Could you check a few things on this drawing? It's one solid part, dimensions in mm from its lowest x, y, z. A direction names the side the tool comes from. Round coordinates to 2 decimals unless told otherwise and drop trailing zeros. Write each loop counter-clockwise with the first axis right and the second up, starting at its lowest first coordinate (ties: lowest second). Pieces come first, ordered by that corner, then holes. Notation, with made-up numbers: (60, 10.5) -> (92, 10.5) arc R3 cw to (92, 14.5) -> close; hole circle Ø9 at (-19.75, -36). An arc over 180 degrees is marked (long way). Put each result on its own line as item: value. Start each with the question number.
1) Which directions (+Z, -Z, +X, -X, +Y, -Y) give clear straight access to the entire face, cutting with the end or side of a thin tool? Please do the marked faces 1 and 2.
2) I want a section at D-D, the plane y = 8.5. List the corners of the cut face in (x, z) for me (1 decimal).
3) I want a section at A-A, the plane y = 14. List the corners of the cut face in (x, z) for me (1 decimal).
4) If I drill on line 1 along Z through (x, y) = (29, 6.5); line 2 along Z through (x, y) = (22, 17.5) (1 decimal); line 3 along X through (y, z) = (15.5, 23) (1 decimal), over which ranges is the centre line in solid material (lowest first)? Write a range as [from, to].
5) Will these pins go through, and if not, where does the flat tip stop? P1, Ø10, axis at y = 4.5, z = 47.5, coming from the +X side; P2, Ø3, axis at y = 15.5, z = 24.5, coming from the +X side; P3, Ø3, axis at x = 30.5, y = 14.5, coming from the -Z side.
6) We'd pull the mould along Z, two halves only. Please class the marked faces 3, 4 and 5: released by +Z, released by -Z, zero draft, split by the parting line, or undercut.
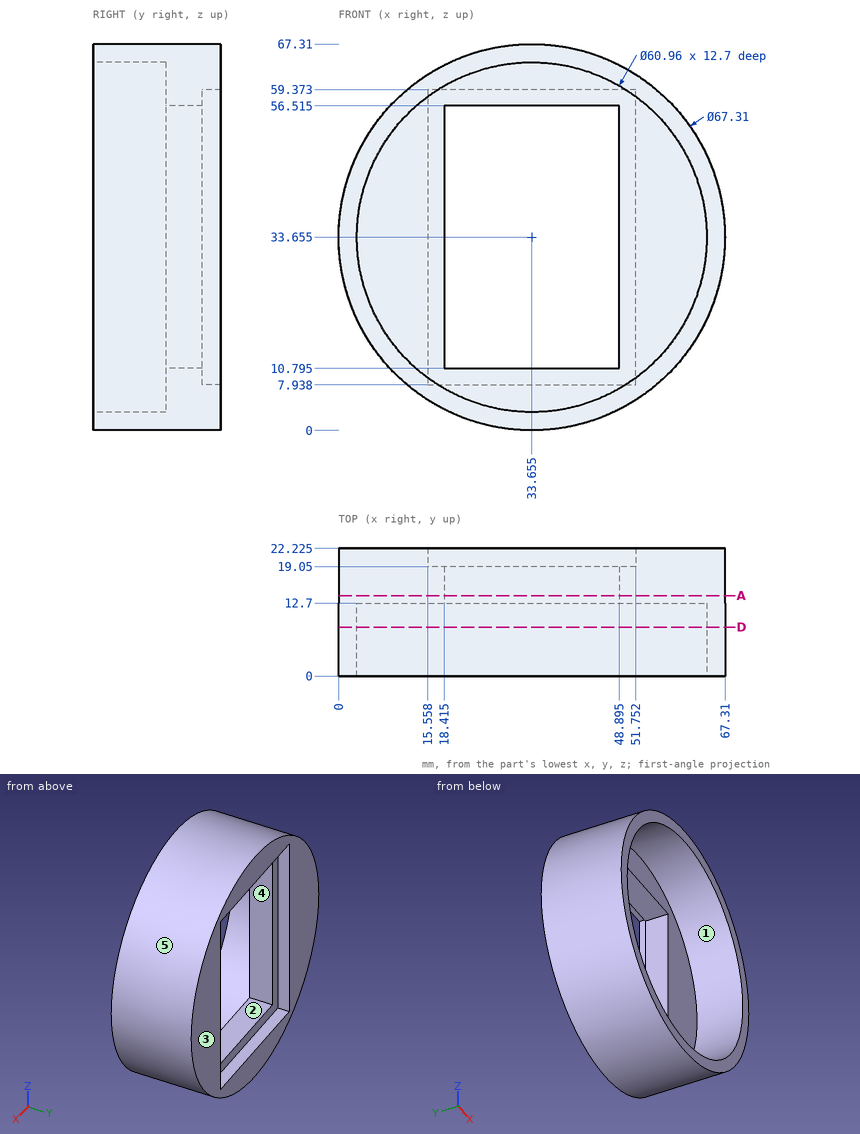
Findings:
1. face 1: -Y
1. face 2: +Y, -Y
2. outline: circle Ø67.3 at (33.7, 33.7); hole circle Ø61 at (33.7, 33.7)
3. outline: circle Ø67.3 at (33.7, 33.7); hole (18.4, 10.8) -> (48.9, 10.8) -> (48.9, 56.5) -> (18.4, 56.5) -> close
4. line 1: z = [0.32, 3.53], [63.78, 66.99]
4. line 2: z = [2.1, 10.8], [56.5, 65.2]
4. line 3: x = [1.7, 18.4], [48.9, 65.6]
5. P1: stops at x = 66.13
5. P2: stops at x = 66.43
5. P3: stops at z = 0.04
6. face 3: zero draft
6. face 4: undercut
6. face 5: split by the parting line
